```python
from build123d import *

# Parameters (mm, degrees)
SKETCH1_W           = 165.1
SKETCH1_H           = 69.85
BOSS_EXTRUDE1_DEPTH = 3
SKETCH3_R           = 2.0828
CUT_EXTRUDE2_DEPTH  = 5.08
SKETCH4_R           = 1.625
CUT_EXTRUDE3_DEPTH  = 17.78


with BuildPart() as part:
    # Sketch1 → Boss-Extrude1 (new body)
    with BuildSketch(Plane(origin=(0, 0, 0), x_dir=(1, 0, 0), z_dir=(0, 1, 0))):
        Rectangle(SKETCH1_W, SKETCH1_H)
    extrude(amount=BOSS_EXTRUDE1_DEPTH)

    # Sketch3 → Cut-Extrude2 (cut)
    with BuildSketch(Plane(origin=(0, 3, 0), x_dir=(1, 0, 0), z_dir=(0, 1, 0))):
        with Locations(Location((-75.692, 0, 0), (0, 0, 270))):
            Circle(SKETCH3_R)
        with Locations(Location((75.692, 0, 0), (0, 0, 270))):
            Circle(SKETCH3_R)
        with Locations(Location((0, -29.337, 0), (0, 0, 270))):
            Circle(SKETCH3_R)
        with Locations(Location((0, 29.337, 0), (0, 0, 270))):
            Circle(SKETCH3_R)
    extrude(amount=-CUT_EXTRUDE2_DEPTH, mode=Mode.SUBTRACT)

    # Sketch4 → Cut-Extrude3 (cut)
    with BuildSketch(Plane(origin=(0, 3, 0), x_dir=(1, 0, 0), z_dir=(0, 1, 0))):
        with Locations(Location((-69.85, 29, 0), (0, 0, 270))):
            Circle(SKETCH4_R)
        with Locations(Location((-46.85, 29, 0), (0, 0, 270))):
            Circle(SKETCH4_R)
        with Locations(Location((-46.85, -29, 0), (0, 0, 270))):
            Circle(SKETCH4_R)
        with Locations(Location((-69.85, -29, 0), (0, 0, 270))):
            Circle(SKETCH4_R)
    extrude(amount=-CUT_EXTRUDE3_DEPTH, mode=Mode.SUBTRACT)


solid = part.part
```
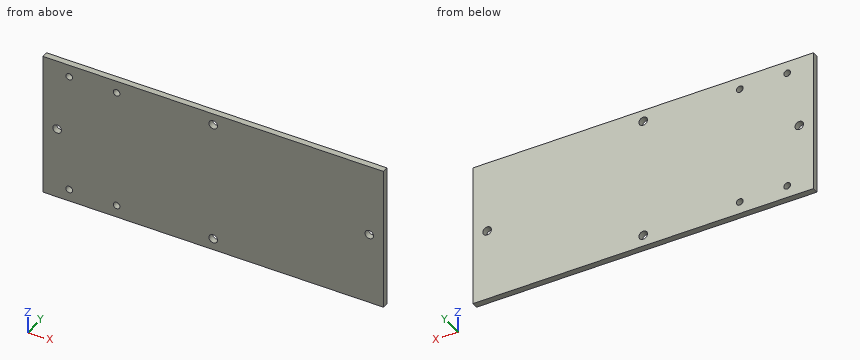
Verification items for the finished model (mm, model axes). Give positions to 0.01 mm unless a question says otherwise; leave off trailing zeros. Loops run counter-clockwise (first coordinate to the right, second up) from the corner with the lowest first, then second, coordinate; pieces in that order, holes last. Notation, with made-up numbers: M 36,-17.5 L 84,-17.5 A21 cw 84,-13.5 Z; hole C -40,67 d7. An arc over 180 degrees is marked long. Return JSON: item names as keys, results as strings.
1) Section check B-B, the plane z = 29. Enter the section's corners in (x, y) (3 decimals).
Findings:
{"outline": "M -82.55,0 L -71.475,0 L -71.475,3 L -82.55,3 Z; M -68.225,0 L -48.475,0 L -48.475,3 L -68.225,3 Z; M -45.225,0 L -2.055,0 L -2.055,3 L -45.225,3 Z; M 2.055,0 L 82.55,0 L 82.55,3 L 2.055,3 Z"}
2) Material ranges on L1, parallel to X at y = 0.6, z = -29 (3 decimals); L2, parallel to X at y = 1, z = -29.5, recorded low to high. Write a range as [from, to].
Findings:
{"L1": "x = [-82.55, -71.475], [-68.225, -48.475], [-45.225, -2.055], [2.055, 82.55]", "L2": "x = [-82.55, -71.4], [-68.3, -48.4], [-45.3, -2.08], [2.08, 82.55]"}
3) Section check A-A, the plane x = 0. Enter the section's corners in (y, z) (3 decimals).
Findings:
{"outline": "M 0,-34.925 L 3,-34.925 L 3,-31.42 L 0,-31.42 Z; M 0,-27.254 L 3,-27.254 L 3,27.254 L 0,27.254 Z; M 0,31.42 L 3,31.42 L 3,34.925 L 0,34.925 Z"}
4) Section check C-C, the plane x = -69.85. Enter the section's corners in (y, z) (3 decimals), and give its area (3 significant figures).
Findings:
{"outline": "M 0,-34.925 L 3,-34.925 L 3,-30.625 L 0,-30.625 Z; M 0,-27.375 L 3,-27.375 L 3,27.375 L 0,27.375 Z; M 0,30.625 L 3,30.625 L 3,34.925 L 0,34.925 Z", "area": "190 mm2"}
